```python
from build123d import *

# Parameters (mm, degrees)
RESSALTO_EXTRUS_O1_DEPTH = 2
ESBO_O2_R                = 4.5
CORTE_EXTRUS_O1_DEPTH    = 2


with BuildPart() as part:
    # Esboço1 → Ressalto-extrusão1 (new body)
    with BuildSketch(Plane(origin=(0, 0, 0), x_dir=(1, 0, 0), z_dir=(0, 1, 0))):
        with BuildLine():
            Line((6, -2.5), (14, -2.5))
            ThreePointArc((14, -2.5), (26.5, 0), (14, 2.5))
            Line((14, 2.5), (6, 2.5))
            ThreePointArc((6, 2.5), (-6.5, 0), (6, -2.5))
        make_face()
    extrude(amount=-RESSALTO_EXTRUS_O1_DEPTH)

    # Esboço2 → Corte-extrusão1 (cut)
    with BuildSketch(Plane(origin=(0, 0, 0), x_dir=(1, 0, 0), z_dir=(0, 1, 0))):
        with Locations(Location((0, 0, 0), (0, 0, 270))):
            Circle(ESBO_O2_R)
        with Locations(Location((20, 0, 0), (0, 0, 270))):
            Circle(ESBO_O2_R)
    extrude(amount=-CORTE_EXTRUS_O1_DEPTH, mode=Mode.SUBTRACT)


solid = part.part
```
The model under review builds one solid part; all positions refer to its coordinate system, in mm. A direction names the side the tool comes from. Give positions to 0.01 mm unless a question says otherwise; leave off trailing zeros. Write each loop counter-clockwise with the first axis right and the second up, starting at its lowest first coordinate (ties: lowest second). Pieces come first, ordered by that corner, then holes. Notation, with made-up numbers: (23, -24) -> (38, -24) arc R30 cw to (38, 6) -> close; hole circle Ø11 at (-19.5, 16). An arc over 180 degrees is marked (long way). Answer in a Markdown table with one row per item.
1) Add section A-A on x = 20. State the section outline as (y, z) points, plus the area to 3 significant figures.
Worked answers:
| item | result |
|---|---|
| outline | (-2, -6.5) -> (0, -6.5) -> (0, -4.5) -> (-2, -4.5) -> close; (-2, 4.5) -> (0, 4.5) -> (0, 6.5) -> (-2, 6.5) -> close |
| area | 8.00 mm² |
2) Add section C-C on z = 0. State the section outline as (x, y) points, plus the area to 3 significant figures.
Worked answers:
| item | result |
|---|---|
| outline | (-6.5, -2) -> (-4.5, -2) -> (-4.5, 0) -> (-6.5, 0) -> close; (4.5, -2) -> (15.5, -2) -> (15.5, 0) -> (4.5, 0) -> close; (24.5, -2) -> (26.5, -2) -> (26.5, 0) -> (24.5, 0) -> close |
| area | 30.0 mm² |
3) Mouldability with a two-part tool opening along Z and no side actions: class faces 1 (the cylindrical face through (24.46, -0.99, -0.59)), 2 (the cylindrical face through (1.352, -0.986, 4.292)), 3 (the flat face through (10, -1, -2.5)), 4 (the flat face through (10, 0, 0)) as +Z half, -Z half, draft (parallel to the pull), parting line (faces both ways), or undercut.
Worked answers:
| item | result |
|---|---|
| face 1 | undercut |
| face 2 | undercut |
| face 3 | -Z half |
| face 4 | draft |
4) For L1, parallel to X at y = -1.9, z = -0.25; L2, parallel to X at y = -0.65, z = 2.75; L3, parallel to X at y = -0.15, z = 1.5, list the stretches that pass through material, from the lowest coordinate up. Write a range as [from, to].
Worked answers:
| item | result |
|---|---|
| L1 | [-6.5, -4.49], [4.49, 15.51], [24.49, 26.5] |
| L2 | [-5.89, -3.56], [3.56, 5.89], [14.11, 16.44], [23.56, 25.89] |
| L3 | [-6.32, -4.24], [4.24, 15.76], [24.24, 26.32] |
5) Add section D-D on z = 4. State the section outline as (x, y) points, plus the area to 3 significant figures.
Worked answers:
| item | result |
|---|---|
| outline | (-5.12, -2) -> (-2.06, -2) -> (-2.06, 0) -> (-5.12, 0) -> close; (2.06, -2) -> (5.12, -2) -> (5.12, 0) -> (2.06, 0) -> close; (14.88, -2) -> (17.94, -2) -> (17.94, 0) -> (14.88, 0) -> close; (22.06, -2) -> (25.12, -2) -> (25.12, 0) -> (22.06, 0) -> close |
| area | 24.5 mm² |
6) Tool access review of faces 5 (the cylindrical face through (26.495, -0.986, 0.25)), 6 (the flat face through (10, -1, 2.5)): name each direction out of +Z, -Z, +X, -X, +Y, -Y from which nothing blocks a thin tool from reaching the whole face with its end or side.
Worked answers:
| item | result |
|---|---|
| face 5 | +Y, -Y |
| face 6 | +Z, +Y, -Y |
7) Add section B-B on y = -1.5. State the section outline as (x, z) points.
Worked answers:
| item | result |
|---|---|
| outline | (6, -2.5) -> (14, -2.5) arc R6.5 ccw (long way) to (14, 2.5) -> (6, 2.5) arc R6.5 ccw (long way) to start; hole circle Ø9 at (0, 0); hole circle Ø9 at (20, 0) |
8) Clearance check with flat-ended pins moving along their axes: P1, Ø1, axis at x = 3.5, z = 0, coming from the -Y side; P2, Ø1, axis at y = -0.5, z = -2, coming from the -X side; P3, Ø1, axis at x = 1.5, y = -0.5, coming from the -Z side. State where each tip first meets the part, or that it passes through.
Worked answers:
| item | result |
|---|---|
| P1 | through |
| P2 | x = -6.32 |
| P3 | z = -6.42 |
